Build history of the part. All positions in model axes, mm. Face numbers are marked on the shaded views. Round coordinates to 2 decimals unless told otherwise and drop trailing zeros. Write each loop counter-clockwise with the first axis right and the second up, starting at its lowest first coordinate (ties: lowest second). Pieces come first, ordered by that corner, then holes. Notation, with made-up numbers: M -3.75,-36 L 19.25,-36 A23 ccw 19.25,-12 Z; hole C 23.5,5 d5. An arc over 180 degrees is marked long. Use a Markdown table: item, result.
from build123d import *

# Parameters (mm, degrees)
SKETCH1_R               = 26
SKETCH1_R_2             = 23.9
BOSS_EXTRUDE1_DEPTH     = 350
SKETCH3_R               = 2.75
CUT_EXTRUDE2_DEPTH      = 352.926128612
CIRPATTERN1_COUNT       = 3
CUT_EXTRUDE3_DEPTH      = 352.926128726
CUT_EXTRUDE3_DEPTH_BACK = 352.926128726
SKETCH5_R               = 2.75
CUT_EXTRUDE4_DEPTH      = 352.926128726
CUT_EXTRUDE4_DEPTH_BACK = 352.926128726
SKETCH6_R               = 2.194915


with BuildPart() as part:
    # Sketch1 → Boss-Extrude1 (new body)
    with BuildSketch(Plane(origin=(0, 0, 0), x_dir=(1, 0, 0), z_dir=(0, 1, 0))):
        with Locations(Location((0, 0, 0), (0, 0, 270))):
            Circle(SKETCH1_R)
        with Locations(Location((0, 0, 0), (0, 0, 270))):
            Circle(SKETCH1_R_2, mode=Mode.SUBTRACT)
    extrude(amount=BOSS_EXTRUDE1_DEPTH)

    # Sketch3 → Cut-Extrude2 (cut, through all)
    with BuildSketch(Plane.XY):
        with Locations(Location((0, 70, 0), (0, 0, 90))):
            Circle(SKETCH3_R)
        with Locations(Location((0, 200, 0), (0, 0, 90))):
            Circle(SKETCH3_R)
    cut_extrude2 = extrude(amount=-CUT_EXTRUDE2_DEPTH, mode=Mode.SUBTRACT)

    # CirPattern1: Cut-Extrude2 ×3 about axis
    cirpattern1_axis = Axis((0, 350, 0), (0, -1, 0))
    for i in range(1, CIRPATTERN1_COUNT):
        add(cut_extrude2.rotate(cirpattern1_axis, i * 360 / CIRPATTERN1_COUNT), mode=Mode.SUBTRACT)

    # Sketch5 → Cut-Extrude3 (cut, two sides: drawn at the far end of the back side and taken through both)
    with BuildSketch(Plane(origin=(0, 0, 0), x_dir=(0, 0, -1), z_dir=(1, 0, 0)).offset(-CUT_EXTRUDE3_DEPTH_BACK)):
        with Locations((0, 200)):
            Circle(SKETCH5_R)
        with Locations((0, 70)):
            Circle(SKETCH5_R)
    extrude(amount=CUT_EXTRUDE3_DEPTH + CUT_EXTRUDE3_DEPTH_BACK, mode=Mode.SUBTRACT)

    # Sketch6 → Cut-Extrude4 (cut, two sides: drawn at the far end of the back side and taken through both)
    with BuildSketch(Plane.XY.offset(-CUT_EXTRUDE4_DEPTH_BACK)):
        with Locations((0, 342)):
            Circle(SKETCH6_R)
    extrude(amount=CUT_EXTRUDE4_DEPTH + CUT_EXTRUDE4_DEPTH_BACK, mode=Mode.SUBTRACT)


solid = part.part
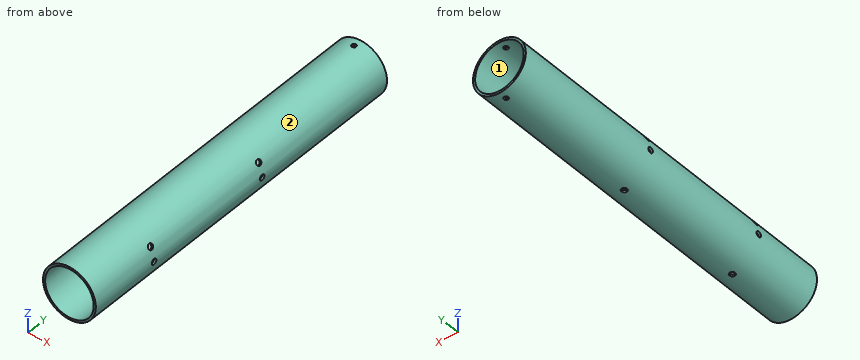
Q1. Drill centre lines: L1, parallel to Y at x = 24.3, z = 0; L2, parallel to Z at x = -0.5, y = 233; L3, parallel to Y at x = 0, z = 24.8. Where is each one in solid material? Low to high.
Response values:
| item | result |
|---|---|
| L1 | y = 0 to 67.25, 72.75 to 197.25, 202.75 to 350 |
| L2 | z = -26 to -23.89, 23.89 to 26 |
| L3 | y = 0 to 339.81, 344.19 to 350 |
Q2. Two-plate mould, pull along X, no slides. Class the marked faces 1 and 2: +X half, -X half, draft (parallel to the pull), parting line (faces both ways), or undercut.
Response values:
| item | result |
|---|---|
| face 1 | undercut |
| face 2 | parting line |
Q3. Cut at B-B on x = -8. Give the cut face in (y, z).
Response values:
| item | result |
|---|---|
| outline | M 0,-24.74 L 350,-24.74 L 350,-22.52 L 0,-22.52 Z; M 0,22.52 L 350,22.52 L 350,24.74 L 0,24.74 Z |
Q4. Drop flat-ended pins along their axis: P1, Ø2.5, axis at x = 0, y = 342, coming from the +Z side; P2, Ø4, axis at y = 54, z = -12, coming from the +X side; P3, Ø1.5, axis at x = 15.5, y = 292, coming from the +Z side; P4, Ø8, axis at y = 40, z = -15.5, coming from the +X side. Give the stop position or say it passes through.
Response values:
| item | result |
|---|---|
| P1 | passes through |
| P2 | stops at x = 24 |
| P3 | stops at z = 21.41 |
| P4 | stops at x = 23.32 |
Q5. Cut at C-C on y = 272. Give the cut face in (x, z), and give its area (3 significant figures).
Response values:
| item | result |
|---|---|
| outline | C 0,0 d52; hole C 0,0 d47.8 |
| area | 329 mm2 |
Q6. Cut at A-A on z = -6.5. Give the cut face in (x, y).
Response values:
| item | result |
|---|---|
| outline | M -25.17,0 L -23,0 L -23,350 L -25.17,350 Z; M 23,0 L 25.17,0 L 25.17,350 L 23,350 Z |
